Could you check a few things on this model? Use its own coordinates, in mm. A direction names the side the tool comes from. Coordinates: 2 decimals unless noted, no trailing zeros. Loops run counter-clockwise (first coordinate to the right, second up) from the corner with the lowest first, then second, coordinate; pieces in that order, holes last. Notation, with made-up numbers: (29, 85) -> (60, 85) arc R8 ccw to (60, 92) -> close; hole circle Ø6 at (25.25, 6). An arc over 180 degrees is marked (long way). One line per question, with ' | ' between items. Start each with the question number.
(1) Suppose I cut it at B-B (x = 2). Please give me the cut outline in (y, z).
(2) Suppose I cut it at D-D (y = -103). Please give me the cut outline in (x, z), plus the area to 3 significant figures.
(3) Suppose I cut it at C-C (z = 60). Please give me the cut outline in (x, y), plus the area to 3 significant figures.
(4) If I drill on line 1 along Z through (x, y) = (1.9, -79); line 2 along Z through (x, y) = (0.85, 21); line 3 along Y through (x, z) = (3.75, 34), over which ranges is the centre line in solid material (lowest first)?
(5) If we mould it in two halves opening along Z, with no side actions, what happens to faces 4 (the face through (2, -70, 5.678)), 5 (the face through (0, -28, 25)), 6 (the face through (2.535, 6.749, 24.225))? For each: pulls with the +Z half, pulls with the -Z half, needs draft (parallel to the pull), parting line crosses it, or undercut.
(6) I'm going to push flat-ended pins straight in: pin 1 Ø2.5 at (x, z) = (3.5, -8.5) entering from -Y; pin 2 Ø2.5 at (x, y) = (3, -51) entering from -Z. Where does each tip first touch, or does it pass through?
(7) Which directions (+Z, -Z, +X, -X, +Y, -Y) give clear straight access to the entire face, cutting with the end or side of a thin tool? Please do faces 1 (the face through (2, -18.967, 65)), 2 (the face through (2, -18.967, -10)), 3 (the face through (2, 31.033, 24)).
(8) Suppose I cut it at A-A (y = 3). Please give me the cut outline in (x, z).
```python
from build123d import *

# Parameters (mm, degrees)
F1_DEPTH = 5
F2_D     = 8.5
F3_D     = 11


# Not quite as in the source:
# - a feature names something its author has since deleted; it is built from what else it names


with BuildPart() as f1:
    # F0 (on Right) → F1 (new body)
    with BuildSketch(Plane.YZ):
        Polygon((31.0329496861, 74.6778247207), (-18.9670503139, 74.6778247207), (-18.9670503139, 55.6778247207), (-118.9670503139, 55.6778247207), (-118.9670503139, 5.6778247207), (-18.9670503139, 5.6778247207), (-18.9670503139, -25.3221752793), (31.0329496861, -25.3221752793), align=None)
    extrude(amount=F1_DEPTH)

    # F2 (through all)
    with Locations(Plane(origin=(0, 0, 0), x_dir=(0, 1, 0), z_dir=(-1, 0, 0))):
        with Locations((-8.9670503139, -67.6778247207), (21.0329496861, -67.6778247207)):
            Hole(F2_D / 2)

    # F3 (through all)
    with Locations(Plane(origin=(0, 0, 0), x_dir=(0, 1, 0), z_dir=(-1, 0, 0))):
        with Locations((6.0329496861, -29.6778247207), (6.0329496861, 10.3221752793), (-93.9670503139, -30.6778247207)):
            Hole(F3_D / 2)


solid = f1.part
```
Checks:
1) outline: (-118.97, 5.68) -> (-18.97, 5.68) -> (-18.97, -25.32) -> (31.03, -25.32) -> (31.03, 74.68) -> (-18.97, 74.68) -> (-18.97, 55.68) -> (-118.97, 55.68) -> close; hole circle Ø11 at (-93.97, 30.68); hole circle Ø8.5 at (-8.97, 67.68); hole circle Ø11 at (6.03, -10.32); hole circle Ø11 at (6.03, 29.68); hole circle Ø8.5 at (21.03, 67.68)
2) outline: (0, 5.68) -> (5, 5.68) -> (5, 55.68) -> (0, 55.68) -> close | area: 250 mm^2
3) outline: (0, -18.97) -> (5, -18.97) -> (5, 31.03) -> (0, 31.03) -> close | area: 250 mm^2
4) line 1: z = 5.68 to 55.68 | line 2: z = -25.32 to 63.43, 71.93 to 74.68 | line 3: y = -118.97 to -98.35, -89.58 to 2.63, 9.43 to 31.03
5) face 4: pulls with the -Z half | face 5: needs draft | face 6: undercut
6) pin 1: stops at y = -18.97 | pin 2: stops at z = 5.68
7) face 1: +Z, +X, -X, -Y | face 2: -Z, +X, -X, -Y | face 3: +Z, -Z, +X, -X, +Y
8) outline: (0, -25.32) -> (5, -25.32) -> (5, -14.91) -> (0, -14.91) -> close; (0, -5.73) -> (5, -5.73) -> (5, 25.09) -> (0, 25.09) -> close; (0, 34.27) -> (5, 34.27) -> (5, 74.68) -> (0, 74.68) -> close
